Design review of the part shown in the three views and the two pictorial views. Dimensions are in mm from the part's minimum x, y and z. A direction names the side the tool comes from. Give positions to 0.01 mm unless a question says otherwise; leave off trailing zeros. Order: outer loops, then holes, each group sorted by start corner. A loop starts at its lowest first (then second) coordinate and runs counter-clockwise, first axis right, second up.
Item 1: Machinability: for the marked faces 1, 2 and 3, which of the approach directions +Z, -Z, +X, -X, +Y, -Y give a long, thin tool a straight path to every point of the face, cutting with its end or side? Answer none if there is none.
Item 2: Consider section B-B (y = 10.25). Give the boundary of the cut face in (x, z).
Item 3: For probe 1 along X at (y, z) = (10.25, 18) (1 decimal); probe 2 along X at (y, z) = (11.5, 25); probe 3 along Y at (x, z) = (38.5, 29.5), list the stretches that pass through material, from the lowest coordinate up.
Item 4: Consider section D-D (y = 14.25). Give the boundary of the cut face in (x, z).
Item 5: Consider section C-C (x = 13). Give the boundary of the cut face in (y, z) (1 decimal), plus the area to 3 significant figures.
Item 6: The part is to be moulded in two halves that separate along X. For the marked faces 4, 5 and 6, say which applies: released by +X, released by -X, zero draft, split by the parting line, or undercut.
Item 7: Consider section A-A (z = 27). Give the boundary of the cut face in (x, y) (1 decimal).
Item 8: For P1, Ø9, axis at y = 10, z = 18, coming from the +X side; P2, Ø1, axis at x = 11.5, z = 22.5, coming from the +Y side; P3, Ø7.5, axis at x = 10.5, z = 21, coming from the +Y side, all flat-tipped, find the tip position at first contact; note any pin that passes through.
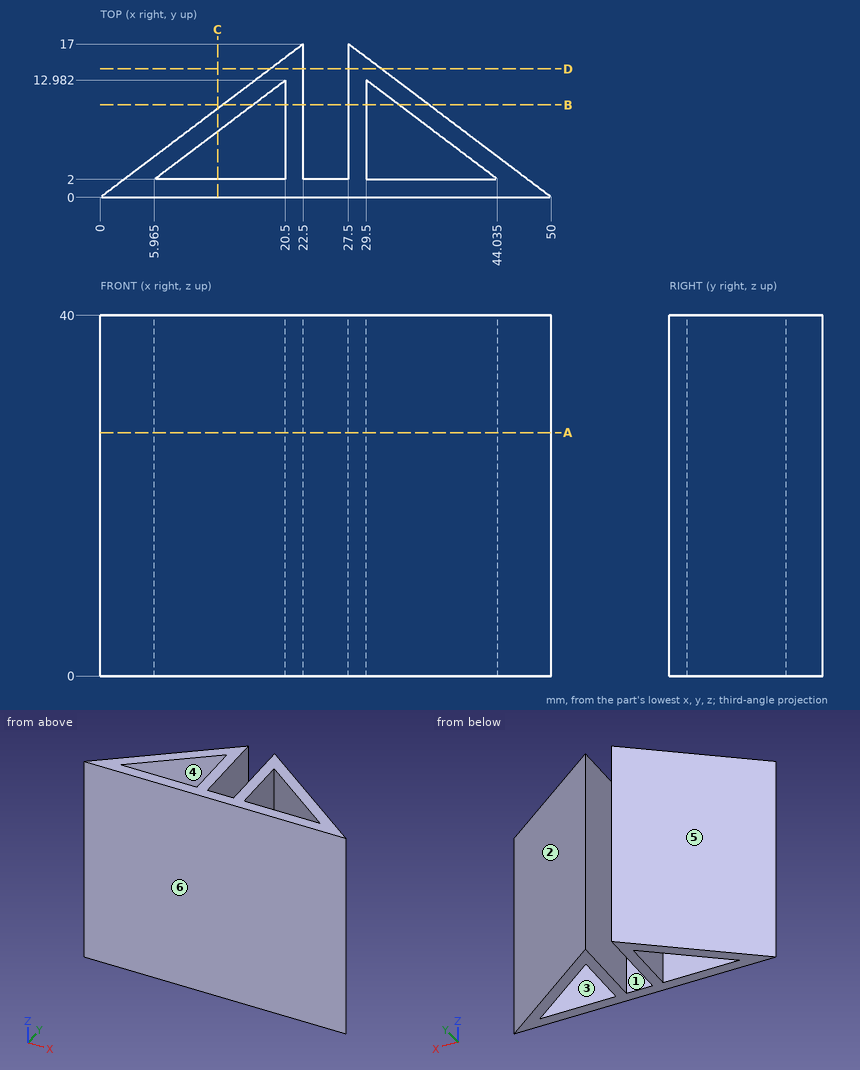
Resolved:
1. face 1: +Z, -Z, +Y
1. face 2: +Z, -Z, +X, +Y
1. face 3: +Z, -Z
2. outline: (13.57, 0) - (16.88, 0) - (16.88, 40) - (13.57, 40) - close; (20.5, 0) - (22.5, 0) - (22.5, 40) - (20.5, 40) - close; (27.5, 0) - (29.5, 0) - (29.5, 40) - (27.5, 40) - close; (33.12, 0) - (36.43, 0) - (36.43, 40) - (33.12, 40) - close
3. probe 1: x = 13.6 to 16.9, 20.5 to 22.5, 27.5 to 29.5, 33.1 to 36.4
3. probe 2: x = 15.22 to 18.54, 20.5 to 22.5, 27.5 to 29.5, 31.46 to 34.78
3. probe 3: y = 0 to 2, 6.18 to 8.69
4. outline: (18.86, 0) - (22.5, 0) - (22.5, 40) - (18.86, 40) - close; (27.5, 0) - (31.14, 0) - (31.14, 40) - (27.5, 40) - close
5. outline: (0, 0) - (2, 0) - (2, 40) - (0, 40) - close; (7.3, 0) - (9.8, 0) - (9.8, 40) - (7.3, 40) - close
5. area: 180 mm2
6. face 4: undercut
6. face 5: released by -X
6. face 6: zero draft
7. outline: (0, 0) - (50, 0) - (27.5, 17) - (27.5, 2) - (22.5, 2) - (22.5, 17) - close; hole (6, 2) - (20.5, 2) - (20.5, 13) - close; hole (29.5, 2) - (44, 2) - (29.5, 13) - close
8. P1: stops at x = 42.72
8. P2: stops at y = 9.07
8. P3: stops at y = 10.77
